Build history of the part. All positions in model axes, mm. A direction names the side the tool comes from. Round coordinates to 2 decimals unless told otherwise and drop trailing zeros. Loops run counter-clockwise (first coordinate to the right, second up) from the corner with the lowest first, then second, coordinate; pieces in that order, holes last. Notation, with made-up numbers: M -30,76.5 L -23,76.5 A15 ccw -23,93.5 Z; hole C 64,71.25 d3. An arc over 180 degrees is marked long. One line per item, written item: value.
```python
from build123d import *

# Parameters (mm, degrees)
SKETCH1_R           = 12
SKETCH1_R_2         = 1.5
BOSS_EXTRUDE1_DEPTH = 2.5
BOSS_EXTRUDE2_DEPTH = 2.5
SKETCH3_W           = 50
SKETCH3_H           = 2.5
BOSS_EXTRUDE3_DEPTH = 30
SKETCH4_W           = 5
SKETCH4_H           = 18
CUT_EXTRUDE1_DEPTH  = 3.5
BOSS_EXTRUDE4_DEPTH = 3
CHAMFER1_SIZE       = 1


with BuildPart() as part:
    # Sketch1 → Boss-Extrude1 (new body)
    with BuildSketch(Plane.XY):
        Polygon((25, 18.15), (22, 21.15), (-22, 21.15), (-25, 18.15), (-25, -23.85), (-22, -26.85), (22, -26.85), (25, -23.85), align=None)
        Circle(SKETCH1_R, mode=Mode.SUBTRACT)
        with Locations((-15.5, 15.5)):
            Circle(SKETCH1_R_2, mode=Mode.SUBTRACT)
        with Locations((15.5, 15.5)):
            Circle(SKETCH1_R_2, mode=Mode.SUBTRACT)
        with Locations((-15.5, -15.5)):
            Circle(SKETCH1_R_2, mode=Mode.SUBTRACT)
        with Locations((15.5, -15.5)):
            Circle(SKETCH1_R_2, mode=Mode.SUBTRACT)
    extrude(amount=BOSS_EXTRUDE1_DEPTH)

    # Sketch2 → Boss-Extrude2 (add)
    with BuildSketch(Plane(origin=(0, 0, 0), x_dir=(-1, 0, 0), z_dir=(0, 0, -1))):
        Polygon((-25, -23.85), (-25, -29.85), (25, -29.85), (25, -23.85), (22, -26.85), (-22, -26.85), align=None)
    extrude(amount=-BOSS_EXTRUDE2_DEPTH)

    # Sketch3 → Boss-Extrude3 (add)
    with BuildSketch(Plane.XY.offset(2.5)):
        with Locations((0, -28.6)):
            Rectangle(SKETCH3_W, SKETCH3_H)
    extrude(amount=BOSS_EXTRUDE3_DEPTH)

    # Sketch4 → Cut-Extrude1 (cut, through all)
    with BuildSketch(Plane(origin=(0, -27.35, 0), x_dir=(1, 0, 0), z_dir=(0, 1, 0))):
        with BuildLine():
            Line((13.5, -29.5), (18.5, -29.5))
            ThreePointArc((18.5, -29.5), (16, -32), (13.5, -29.5))
        make_face()
        with Locations((16, -20.5)):
            Rectangle(SKETCH4_W, SKETCH4_H)
        with BuildLine():
            Line((13.5, -11.5), (18.5, -11.5))
            ThreePointArc((18.5, -11.5), (16, -9), (13.5, -11.5))
        make_face()
        with BuildLine():
            Line((-18.5, -11.5), (-13.5, -11.5))
            ThreePointArc((-13.5, -11.5), (-16, -9), (-18.5, -11.5))
        make_face()
        with Locations((-16, -20.5)):
            Rectangle(SKETCH4_W, SKETCH4_H)
        with BuildLine():
            ThreePointArc((-13.5, -29.5), (-16, -32), (-18.5, -29.5))
            Line((-18.5, -29.5), (-13.5, -29.5))
        make_face()
    extrude(amount=-CUT_EXTRUDE1_DEPTH, mode=Mode.SUBTRACT)

    # Sketch5 → Boss-Extrude4 (add)
    with BuildSketch(Plane(origin=(25, 0, 0), x_dir=(0, 0, -1), z_dir=(1, 0, 0))):
        Polygon((-2.5, -27.35), (-2.5, -20.278932188), (-9.571067812, -27.35), align=None)
    boss_extrude4 = extrude(amount=-BOSS_EXTRUDE4_DEPTH)

    # Mirror1: Boss-Extrude4 across plane
    add(boss_extrude4.mirror(Plane(origin=(0, 0, 0), x_dir=(0, 0, 1), z_dir=(1, 0, 0))))

    # Chamfer1
    chamfer1_edges = [part.edges().sort_by_distance(p)[0] for p in [
        (0, -29.85, 0),
    ]]
    chamfer(chamfer1_edges, length=CHAMFER1_SIZE)


solid = part.part
```
Item 1: Wall check: line 1 along Y through (x, z) = (15.5, 1.15); line 2 along Y through (x, z) = (0, 1); line 3 along Y through (x, z) = (-15, 1). Give the ranges that are in metal, low to high.
Check values:
line 1: y = -29.85 to -17, -14 to 14, 17 to 21.15
line 2: y = -29.85 to -12, 12 to 21.15
line 3: y = -29.85 to -16.91, -14.09 to 14.09, 16.91 to 21.15
Item 2: Pull direction Y, two halves, no side cores. Call faces 1 (the face through (-17, 15.57, 1.23)), 2 (the face through (-16, -29, 9)), 3 (the face through (0, -27.35, 17)): pulls with the +Y half, pulls with the -Y half, needs draft (parallel to the pull), parting line crosses it, or undercut.
Check values:
face 1: undercut
face 2: needs draft
face 3: pulls with the +Y half
Item 3: Slice it at C-C, the plane y = -9. Give the cut face in (x, z), and give its area (3 significant figures).
Check values:
outline: M -25,0 L -7.94,0 L -7.94,2.5 L -25,2.5 Z; M 7.94,0 L 25,0 L 25,2.5 L 7.94,2.5 Z
area: 85.3 mm2
Item 4: Which spindle directions (+Z, -Z, +X, -X, +Y, -Y) get a long thin tool onto all of the face, cutting with end or side? Do faces 4 (the face through (-23.521, -23.765, 5.986)), 5 (the face through (22, -25, 5)), 6 (the face through (13.5, -29, 21)). Say none if no direction does.
Check values:
face 4: +Z, +X, -X, +Y
face 5: +Z, +Y
face 6: +Y, -Y
Item 5: Slice it at A-A, the plane x = 0. Give the cut face in (y, z).
Check values:
outline: M -29.85,1 L -28.85,0 L -12,0 L -12,2.5 L -27.35,2.5 L -27.35,32.5 L -29.85,32.5 Z; M 12,0 L 21.15,0 L 21.15,2.5 L 12,2.5 Z
Item 6: Drop flat-ended pins along their axis: P1, Ø1.8, axis at x = -15.5, y = -15.5, coming from the +Z side; P2, Ø3.5, axis at x = 15.5, y = 15.5, coming from the +Z side; P3, Ø5, axis at x = 2, z = 14.5, coming from the +Y side. Give the stop position or say it passes through.
Check values:
P1: passes through
P2: stops at z = 2.5
P3: stops at y = -27.35
Item 7: Slice it at B-B, the plane z = 25. Give the cut face in (x, y), and give its area (3 significant figures).
Check values:
outline: M -25,-29.85 L -18.5,-29.85 L -18.5,-27.35 L -25,-27.35 Z; M -13.5,-29.85 L 13.5,-29.85 L 13.5,-27.35 L -13.5,-27.35 Z; M 18.5,-29.85 L 25,-29.85 L 25,-27.35 L 18.5,-27.35 Z
area: 100 mm2
Item 8: Slice it at D-D, the plane x = 16. Give the cut face in (y, z).
Check values:
outline: M -29.85,1 L -28.85,0 L -16.91,0 L -16.91,2.5 L -27.35,2.5 L -27.35,9 L -29.85,9 Z; M -29.85,32 L -27.35,32 L -27.35,32.5 L -29.85,32.5 Z; M -14.09,0 L 14.09,0 L 14.09,2.5 L -14.09,2.5 Z; M 16.91,0 L 21.15,0 L 21.15,2.5 L 16.91,2.5 Z
